Could you check a few things on this model? Use its own coordinates, in mm. A direction names the side the tool comes from. Round coordinates to 2 decimals unless told otherwise and drop trailing zeros. Loops run counter-clockwise (first coordinate to the right, second up) from the corner with the lowest first, then second, coordinate; pieces in that order, holes last. Notation, with made-up numbers: M 84,-30 L 107,-30 A35 cw 107,8 Z; hole C 17.5,33.25 d8. An arc over 180 degrees is marked long. One line per item, written item: value. Start each with the question number.
Q1. I'm going to push flat-ended pins straight in: pin 1 Ø2 at (x, z) = (-10.5, -25) entering from +Y; pin 2 Ø16.5 at (x, z) = (-339.725, -19.05) entering from +Y; pin 3 Ø3 at (y, z) = (-20, 18.5) entering from -X; pin 4 Ø11.5 at (x, z) = (-339.725, 19.05) entering from +Y. Where does each tip first touch, or does it pass through?
Q2. Please list where these lines run through material, in increasing order: line 1 along X through (y, z) = (-64.5, 19.05) (3 decimals); line 2 along X through (y, z) = (-31, 36); line 3 along X through (y, z) = (-77, 14).
Q3. Imagine slicing it at B-B (y = -19.5). Please give me the cut outline in (x, z).
Q4. Imagine slicing it at A-A (z = -19.05). Please give me the cut outline in (x, y) (3 decimals).
Q5. Which directions (+Z, -Z, +X, -X, +Y, -Y) give clear straight access to the entire face, cutting with the end or side of a thin tool? Please do faces 4 (the face through (-340, -44.45, 1)), 5 (the face through (339, -44.45, 1)), 6 (the face through (345.59, -66.36, 16.62)).
Q6. Thinking about a two-plate mould opening in X: for faces 1 (the face through (345.59, -66.36, -21.48)), 2 (the face through (-5, -44, -44.45)), 3 (the face through (317.5, -23, 1)), which applies, released by +X, released by -X, zero draft, split by the parting line, or undercut?
from build123d import *

# Parameters (mm, degrees)
F0_W     = 723.9
F0_H     = 88.9
F0_R     = 6.35
F1_DEPTH = 88.9
F2_W     = 44.45
F2_H     = 44.45
F3_DEPTH = 101.6


with BuildPart() as f1:
    # F0 (on Front) → F1 (new body)
    with BuildSketch(Plane.XZ):
        Rectangle(F0_W, F0_H)
        with Locations((-339.725, -19.05)):
            Circle(F0_R, mode=Mode.SUBTRACT)
        with Locations((339.725, -19.05)):
            Circle(F0_R, mode=Mode.SUBTRACT)
        with Locations((-339.725, 19.05)):
            Circle(F0_R, mode=Mode.SUBTRACT)
        with Locations((339.725, 19.05)):
            Circle(F0_R, mode=Mode.SUBTRACT)
    extrude(amount=F1_DEPTH)

    # F2 (on face) → F3 (cut)
    with BuildSketch(Plane.XY.offset(44.45)):
        with Locations((-339.725, -22.225)):
            Rectangle(F2_W, F2_H)
        with Locations((339.725, -22.225)):
            Rectangle(F2_W, F2_H)
    extrude(amount=-F3_DEPTH, mode=Mode.SUBTRACT)


solid = f1.part
Report:
1. pin 1: stops at y = 0
1. pin 2: stops at y = -44.45
1. pin 3: stops at x = -317.5
1. pin 4: passes through
2. line 1: x = -361.95 to -346.075, -333.375 to 333.375, 346.075 to 361.95
2. line 2: x = -317.5 to 317.5
2. line 3: x = -361.95 to -343.57, -335.88 to 335.88, 343.57 to 361.95
3. outline: M -317.5,-44.45 L 317.5,-44.45 L 317.5,44.45 L -317.5,44.45 Z
4. outline: M -361.95,-88.9 L -346.075,-88.9 L -346.075,-44.45 L -361.95,-44.45 Z; M -333.375,-88.9 L 333.375,-88.9 L 333.375,-44.45 L 317.5,-44.45 L 317.5,0 L -317.5,0 L -317.5,-44.45 L -333.375,-44.45 Z; M 346.075,-88.9 L 361.95,-88.9 L 361.95,-44.45 L 346.075,-44.45 Z
5. face 4: +Z, -Z, -X, +Y
5. face 5: +Z, -Z, +X, +Y
5. face 6: +Y, -Y
6. face 1: undercut
6. face 2: zero draft
6. face 3: released by +X
